Autodesk Inventor part; units mm, degrees
ref_plane "YZ Plane" through (0, 0, 0) normal (1, 0, 0) x (0, 1, 0)
ref_plane "XZ Plane" through (0, 0, 0) normal (0, 1, 0) x (-1, 0, 0)
ref_plane "XY Plane" through (0, 0, 0) normal (0, 0, 1) x (1, 0, 0)
sketch "Sketch1" plane through (0, 0, 0) normal (0, 1, 0) x (-1, 0, 0)
  line L0 (-41.2899, 41.3823) -> (30.4199, 41.3823)
  line L1 (36.2591, 28.6823) -> (36.2591, -55.3155)
  line L2 (30.4199, -68.0155) -> (-41.2899, -68.0155)
  line L3 (-47.1291, -55.3155) -> (-47.1291, 28.6823)
  line L4 (-47.1291, 28.6823) -> (36.2591, 28.6823)
  line L5 (-47.1291, -55.3155) -> (36.2591, -55.3155)
  line L6 (36.2591, -55.3155) -> (33.4867, -65.6622)
  line L7 (-47.1291, -55.3155) -> (-44.3567, -65.6622)
  line L8 (-47.1291, 28.6823) -> (-44.3567, 39.0291)
  line L9 (36.2591, 28.6823) -> (33.4867, 39.0291)
  arc A0 (-44.3567, -65.6622) -> (-41.2899, -68.0155) centre (-41.2899, -64.8405) ccw
  arc A1 (30.4199, -68.0155) -> (33.4867, -65.6622) centre (30.4199, -64.8405) ccw
  arc A2 (33.4867, 39.0291) -> (30.4199, 41.3823) centre (30.4199, 38.2073) ccw
  arc A3 (-41.2899, 41.3823) -> (-44.3567, 39.0291) centre (-41.2899, 38.2073) ccw
  circle A4 centre (-35.4324, -61.0051) radius 2.5019
  circle A5 centre (24.5624, -61.0051) radius 2.5019
  circle A6 centre (-35.4324, 34.3719) radius 2.5019
  circle A7 centre (24.5624, 34.3719) radius 2.5019
  line L10 (-5.435, 41.3823) -> (-5.435, -68.0155) construction
  circle A8 centre (-5.435, 34.3719) radius 2.5019
  circle A9 centre (-5.435, -61.0051) radius 2.5019
  point P0 (0, 0)
  dimension "d2" = 12.7
  dimension "d3" = 12.7
  dimension "d4" = 15
  dimension "d5" = 15
  dimension "d6" = 15
  dimension "d7" = 83.3882
  dimension "d8" = 109.3978
  dimension "d9" = 3.175
  dimension "d10" = 7.0104
  dimension "d11" = 7.0104
  dimension "d12" = 7.0104
  dimension "d13" = 7.0104
  dimension "d14" = 59.9948
  dimension "d15" = 59.9948
  dimension "d16" = 5.0038
  dimension "d17" = 5.0038
  dimension "d18" = 5.0038
  dimension "d19" = 5.0038
  dimension "d20" = 29.9974
  dimension "d21" = 29.9974
  dimension "d42" = 5.0038
  dimension "d43" = 5.0038
extrude "Extrusion1" add sketch "Sketch1" along normal blind 5.9944
sketch "Sketch2" plane through (0, 5.9944, 0) normal (0, 1, 0) x (1, 0, 0)
  line L0 (47.1291, -28.6823) -> (47.1291, 55.3155)
  line L1 (41.2899, 68.0155) -> (-30.4199, 68.0155)
  line L2 (-36.2591, 55.3155) -> (-36.2591, -28.6823)
  line L3 (-33.0841, 53.9185) -> (43.9541, 53.9185)
  line L4 (47.1291, 50.7435) -> (47.1291, -24.0849)
  line L5 (43.9541, -27.2599) -> (-33.0841, -27.2599)
  line L6 (-36.2591, -24.0849) -> (-36.2591, 50.7435)
  arc A0 (-36.2591, -24.0849) -> (-33.0841, -27.2599) centre (-33.0841, -24.0849) ccw
  arc A1 (43.9541, -27.2599) -> (47.1291, -24.0849) centre (43.9541, -24.0849) ccw
  arc A2 (47.1291, 50.7435) -> (43.9541, 53.9185) centre (43.9541, 50.7435) ccw
  arc A3 (-33.0841, 53.9185) -> (-36.2591, 50.7435) centre (-33.0841, 50.7435) ccw
  point P0 (0, 0)
  point P1 (-36.2591, 53.9185)
  point P2 (47.1291, -27.2599)
  dimension "d25" = 81.1784
  dimension "d26" = 14.097
  dimension "d27" = 3.175
extrude "Extrusion2" add sketch "Sketch2" along normal blind 35.5092
sketch "Sketch3" plane through (0, 41.5036, 0) normal (0, 1, 0) x (1, 0, 0)
  line L0 (-36.2591, 50.7435) -> (-36.2591, -24.0849)
  line L1 (43.9541, 53.9185) -> (-33.0841, 53.9185)
  line L2 (43.1159, 26.9945) -> (43.1159, -0.3359)
  line L3 (-32.2459, -0.3359) -> (-32.2459, 26.9945)
  line L4 (-19.5713, 50.0069) -> (30.4413, 50.0069)
  line L5 (30.4413, -23.3483) -> (-19.5713, -23.3483)
  arc A0 (33.6163, 46.8319) -> (30.4413, 50.0069) centre (30.4413, 46.8319) ccw
  arc A1 (-19.5713, 50.0069) -> (-22.7463, 46.8319) centre (-19.5713, 46.8319) ccw
  arc A2 (-22.7463, -20.1733) -> (-19.5713, -23.3483) centre (-19.5713, -20.1733) ccw
  arc A3 (30.4413, -23.3483) -> (33.6163, -20.1733) centre (30.4413, -20.1733) ccw
  arc A4 (-32.2459, -0.3359) -> (-29.0709, -3.5109) centre (-29.0709, -0.3359) ccw
  arc A5 (-29.0709, 30.1695) -> (-32.2459, 26.9945) centre (-29.0709, 26.9945) ccw
  arc A6 (43.1159, 26.9945) -> (39.9409, 30.1695) centre (39.9409, 26.9945) ccw
  arc A7 (39.9409, -3.5109) -> (43.1159, -0.3359) centre (39.9409, -0.3359) ccw
  line L6 (33.6163, 46.8319) -> (33.6163, 36.5195)
  line L7 (33.6163, -9.8609) -> (33.6163, -20.1733)
  line L8 (-22.7463, -20.1733) -> (-22.7463, -9.8609)
  line L9 (-22.7463, 36.5195) -> (-22.7463, 46.8319)
  line L10 (39.9409, -3.5109) -> (39.9663, -3.5109)
  line L11 (-29.0963, -3.5109) -> (-29.0709, -3.5109)
  line L12 (-29.0709, 30.1695) -> (-29.0963, 30.1695)
  line L13 (39.9663, 30.1695) -> (39.9409, 30.1695)
  arc A8 (39.9663, -3.5109) -> (33.6163, -9.8609) centre (39.9663, -9.8609) ccw
  arc A9 (33.6163, 36.5195) -> (39.9663, 30.1695) centre (39.9663, 36.5195) ccw
  arc A10 (-29.0963, 30.1695) -> (-22.7463, 36.5195) centre (-29.0963, 36.5195) ccw
  arc A11 (-22.7463, -9.8609) -> (-29.0963, -3.5109) centre (-29.0963, -9.8609) ccw
  point P0 (0, 0)
  point P1 (43.1159, -3.5109)
  point P2 (43.1159, 30.1695)
  point P3 (-32.2459, -3.5109)
  point P4 (-22.7463, 50.0069)
  point P5 (33.6163, -23.3483)
  point P6 (33.6163, 50.0069)
  dimension "d30" = 56.3626
  dimension "d31" = 33.6804
  dimension "d32" = 73.3552
  dimension "d35" = 75.3618
  dimension "d36" = 4.0132
  dimension "d37" = 3.9116
  dimension "d38" = 3.175
  dimension "d39" = 6.35
extrude "Extrusion3" cut sketch "Sketch3" against normal blind 35.5092
properties part number "NEAMBox"
Check sheet for the modelled part. Datum: model origin and axes. Units: mm. A direction names the side the tool comes from. Round coordinates to 2 decimals unless told otherwise and drop trailing zeros. Order: outer loops, then holes, each group sorted by start corner. A loop starts at its lowest first (then second) coordinate and runs counter-clockwise, first axis right, second up. Notation, with made-up numbers: M -29,61 L -15,61 A16 cw -15,85 Z; hole C 10.25,23 d8. An arc over 180 degrees is marked long. One line per item, written item: value. Start each with the question number.
1. Access from +Z, -Z, +X, -X, +Y, -Y to the whole of each face (thin tool, end or side, straight path). Record for faces 1 (the flat face through (5, 5.994, -14)), 2 (the flat face through (6, 24, 27.26)), 3 (the cylindrical face through (46.174, 23.5, -53.013)).
2. Section check B-B on z = -14. Enter the section's corners in (x, y), and give its area (3 significant figures).
3. Gauge pin test, flat ends, axial feed: P1, Ø14, axis at x = 11.5, z = 30, coming from the +Y side; P2, Ø10.5, axis at x = 15.5, y = 31.5, coming from the -Z side; P3, Ø18, axis at x = -3.5, y = 21, coming from the +Z side; P4, Ø4.5, axis at x = -24.56, z = 34.37, coming from the +Y side. Record the tip position at first contact, or that the pin passes through.
4. Section check C-C on x = 19.5. Enter the section's corners in (y, z), and give its area (3 significant figures).
5. Release check for a two-part mould opening along Z. For faces 4 (the cylindrical face through (46.22, 23.5, 26.31)), 5 (the cylindrical face through (-35.354, 23.5, -52.964)), 6 (the cylindrical face through (32.711, 23.998, -49.052)) record: released by +Z, released by -Z, zero draft, split by the parting line, or undercut.
6. Scan lines: line 1 along X through (y, z) = (6.5, -14.5); line 2 along Z through (x, y) = (-16.5, 22.5); line 3 along X through (y, z) = (31.5, -46). Record each from-to range of solid material in increasing order.
7. Section check D-D on y = 4.5. Give the number of separate pieces and of enclosed holes in the cut face, and give its area (3 significant figures).
Results found:
1. face 1: +Y
1. face 2: +Z, +X, -X, +Y
1. face 3: -Z, +X, +Y
2. outline: M -36.26,0 L 47.13,0 L 47.13,41.5 L 43.12,41.5 L 43.12,5.99 L -32.25,5.99 L -32.25,41.5 L -36.26,41.5 Z
2. area: 785 mm^2
3. P1: y = 41.5
3. P2: z = -53.92
3. P3: z = 27.26
3. P4: through
4. outline: M 0,-68.02 L 5.99,-68.02 L 5.99,-53.92 L 41.5,-53.92 L 41.5,-50.01 L 5.99,-50.01 L 5.99,23.35 L 41.5,23.35 L 41.5,27.26 L 5.99,27.26 L 5.99,41.38 L 0,41.38 Z
4. area: 934 mm^2
5. face 4: released by +Z
5. face 5: released by -Z
5. face 6: undercut
6. line 1: -36.26 to -32.25, 43.12 to 47.13
6. line 2: -53.92 to -50.01, 23.35 to 27.26
6. line 3: -36.26 to -22.75, 33.62 to 47.13
7. separate pieces: 1
7. enclosed holes: 6
7. area: 8,910 mm^2
